```python
from build123d import *

# Parameters (mm, degrees)
SKETCH_1_W          = 160
SKETCH_1_H          = 98
EXTRUDE_1_DEPTH     = 38
SKETCH_2_W          = 20
SKETCH_2_H          = 96.5
CUT_EXTRUDE_1_DEPTH = 28
SKETCH_3_W          = 19
SKETCH_3_H          = 67
EXTRUDE_2_DEPTH     = 15
SKETCH_4_W          = 16
SKETCH_4_H          = 96.5
CUT_EXTRUDE_2_DEPTH = 8
CHAMFER_1_SIZE      = 8
CUT_EXTRUDE_3_DEPTH = 10


with BuildPart() as part:
    # 草图1 → 凸台-拉伸1 (new body)
    with BuildSketch(Plane.XY):
        with Locations((80, 49)):
            Rectangle(SKETCH_1_W, SKETCH_1_H)
    extrude(amount=EXTRUDE_1_DEPTH)

    # 草图2 → 切除-拉伸1 (cut)
    with BuildSketch(Plane.XY.offset(38)):
        with Locations((150, 48.25)):
            Rectangle(SKETCH_2_W, SKETCH_2_H)
    extrude(amount=-CUT_EXTRUDE_1_DEPTH, mode=Mode.SUBTRACT)

    # 草图3 → 凸台-拉伸2 (add)
    with BuildSketch(Plane.XY.offset(10)):
        with Locations((149.5, 43.5)):
            Rectangle(SKETCH_3_W, SKETCH_3_H)
    extrude(amount=EXTRUDE_2_DEPTH)

    # 草图4 → 切除-拉伸2 (cut)
    with BuildSketch(Plane.ZY):
        with Locations((30, 48.25)):
            Rectangle(SKETCH_4_W, SKETCH_4_H)
    extrude(amount=-CUT_EXTRUDE_2_DEPTH, mode=Mode.SUBTRACT)

    # 倒角1
    chamfer_1_edges = [part.edges().sort_by_distance(p)[0] for p in [
        (8, 48.25, 22),
    ]]
    chamfer(chamfer_1_edges, length=CHAMFER_1_SIZE - 0.0001)  # a hair under: the kernel refuses the full size

    # 草图5 → 切除-拉伸3 (cut)
    with BuildSketch(Plane.XZ):
        Polygon((0, 22), (8, 30), (8, 1.5), (0, 1.5), align=None)
    extrude(amount=-CUT_EXTRUDE_3_DEPTH, mode=Mode.SUBTRACT)


solid = part.part
```
Work out the finished part from the listing and answer in its coordinate system (mm). A direction names the side the tool comes from. Give positions to 0.01 mm unless a question says otherwise; leave off trailing zeros. Loops run counter-clockwise (first coordinate to the right, second up) from the corner with the lowest first, then second, coordinate; pieces in that order, holes last. Notation, with made-up numbers: (-16, 64.5) -> (31, 64.5) arc R17 ccw to (31, 69.5) -> close; hole circle Ø4 at (31.5, 80.25). An arc over 180 degrees is marked (long way). Use CSV: the item, a comma, the result in double quotes.
1. A tool of negligible diameter and unlimited length cuts with its end or side. For faces 5 (the flat face through (160, 49, 3)), 6 (the flat face through (149, 44, 25)), 7 (the flat face through (8, 34.2, 30.5)), 8 (the flat face through (149, 77, 17)), from which of +Z, -Z, +X, -X, +Y, -Y can it reach the whole face along a straight path? Write none if from no direction.
Found:
face 5,"+Z, -Z, +X, +Y, -Y"
face 6,"+Z, +X, -Y"
face 7,"+Z, -X, -Y"
face 8,"+Z, +X"
2. Flat-ended cylindrical pins translate along their axes: pin 1 Ø22 at (x, z) = (146, 25.5) entering from -Y; pin 2 Ø6 at (y, z) = (54, 22) entering from +X; pin 3 Ø15 at (x, y) = (152.5, 57.5) entering from +Z; pin 4 Ø4.5 at (x, z) = (150, 18) entering from -Y. Find the tip coordinate at first contact, or state that the pin passes through.
Found:
pin 1,"y = 0"
pin 2,"x = 159"
pin 3,"z = 25"
pin 4,"y = 10"
3. Straight lines are drawn through the part: line 1 (Y direction, x = 152.5, z = 18); line 2 (X direction, y = 31, z = 31); line 3 (X direction, y = 35.5, z = 20.5). For each, find the intervals that lie inside material, in ascending order.
Found:
line 1,"10 to 77, 96.5 to 98"
line 2,"8 to 140"
line 3,"0 to 159"
4. The part is cut by section B-B (x = 144.5). Write down the section's boundary in (y, z).
Found:
outline,"(0, 0) -> (98, 0) -> (98, 38) -> (96.5, 38) -> (96.5, 10) -> (77, 10) -> (77, 25) -> (10, 25) -> (10, 10) -> (0, 10) -> close"
5. The mould has two halves that part along Y. Classify faces 1 (the flat face through (4, 53, 26)), 2 (the flat face through (149, 10, 17)), 3 (the flat face through (159.6, 62.8, 10)), 4 (the flat face through (150, 96.5, 24)): +Y half, -Y half, draft (parallel to the pull), parting line (faces both ways), or undercut.
Found:
face 1,"draft"
face 2,"-Y half"
face 3,"undercut"
face 4,"undercut"
6. The part is cut by section C-C (z = 16). Write down the section's boundary in (x, y).
Found:
outline,"(0, 10) -> (8, 10) -> (8, 0) -> (140, 0) -> (140, 10) -> (159, 10) -> (159, 77) -> (140, 77) -> (140, 96.5) -> (160, 96.5) -> (160, 98) -> (0, 98) -> close"
7. The part is cut by section D-D (y = 7). Write down the section's boundary in (x, z), then the cut area to 3 significant figures.
Found:
outline,"(0, 0) -> (160, 0) -> (160, 10) -> (140, 10) -> (140, 38) -> (8, 38) -> (8, 1.5) -> (0, 1.5) -> close"
area,"5,230 mm^2"
